from build123d import *

# Parameters (mm, degrees)
SKETCH_1_W          = 143
SKETCH_1_H          = 196
SKETCH_1_W_2        = 62
SKETCH_1_H_2        = 142
EXTRUDE_1_DEPTH     = 20
FILLET_1_R          = 12
SKETCH_2_R          = 3
CUT_EXTRUDE_1_DEPTH = 40
SKETCH_3_R          = 5
CUT_EXTRUDE_2_DEPTH = 40


with BuildPart() as part:
    # 草图1 → 凸台-拉伸1 (new, symmetric)
    with BuildSketch(Plane(origin=(0, 0, 0), x_dir=(1, 0, 0), z_dir=(0, 1, 0))):
        Rectangle(SKETCH_1_W, SKETCH_1_H)
        Rectangle(SKETCH_1_W_2, SKETCH_1_H_2, mode=Mode.SUBTRACT)
    extrude(amount=EXTRUDE_1_DEPTH, both=True)

    # 圆角1
    fillet_1_edges = [part.edges().sort_by_distance(p)[0] for p in [
        (-71.5, 0, -98),
        (71.5, 0, -98),
        (71.5, 0, 98),
        (-71.5, 0, 98),
    ]]
    fillet(fillet_1_edges, radius=FILLET_1_R)

    # 草图2 → 切除-拉伸1 (cut)
    with BuildSketch(Plane(origin=(0, 20, 0), x_dir=(1, 0, 0), z_dir=(0, 1, 0))):
        with Locations((-31, 71)):
            Circle(SKETCH_2_R)
        with Locations((31, 71)):
            Circle(SKETCH_2_R)
        with Locations((31, -71)):
            Circle(SKETCH_2_R)
        with Locations((-31, -71)):
            Circle(SKETCH_2_R)
    extrude(amount=-CUT_EXTRUDE_1_DEPTH, mode=Mode.SUBTRACT)

    # 草图3 → 切除-拉伸2 (cut)
    with BuildSketch(Plane(origin=(0, 20, 0), x_dir=(1, 0, 0), z_dir=(0, 1, 0))):
        with Locations((-71.5, 0)):
            Circle(SKETCH_3_R)
        with Locations((71.5, 0)):
            Circle(SKETCH_3_R)
    extrude(amount=-CUT_EXTRUDE_2_DEPTH, mode=Mode.SUBTRACT)


solid = part.part
The listing builds one solid part. Answer for the finished solid, in the listing's coordinates (mm). A direction names the side the tool comes from. Coordinates: 2 decimals unless noted, no trailing zeros. Loops run counter-clockwise (first coordinate to the right, second up) from the corner with the lowest first, then second, coordinate; pieces in that order, holes last. Notation, with made-up numbers: (52.5, 55.5) -> (75.5, 55.5) arc R5 cw to (75.5, 59.5) -> close; hole circle Ø10 at (26.25, 89). An arc over 180 degrees is marked (long way). Write item = value, one per line. Start each with the question number.
1) A cutting plane is placed at C-C (y = 13). Give the vertices of the cut face in (x, z), then the cut area to 3 significant figures.
2) A cutting plane is placed at A-A (z = -51). Give the vertices of the cut face in (x, y), then the cut area to 3 significant figures.
3) A cutting plane is placed at B-B (x = -19). Give the vertices of the cut face in (y, z), then the cut area to 3 significant figures.
4) The mould has two halves that part along X. Classify faces 3 (the face through (66.5, 0.3, -0.1)), 4 (the face through (-68.08, -0.28, -94.39)), 5 (the face through (-33.19, 0.28, 73.05)): released by +X, released by -X, zero draft, split by the parting line, or undercut.
5) A tool of negligible diameter and unlimited length cuts with its end or side. For faces 1 (the face through (-1, 0, -98)), 2 (the face through (0, 0, 71)), from which of +Z, -Z, +X, -X, +Y, -Y can it reach the whole face along a straight path? Write none if from no direction.
6) Straight lines are drawn through the part: line 1 (X direction, y = -3, z = 37.5); line 2 (Z direction, x = -13.5, y = 0); line 3 (Z direction, x = 29, y = 10). For each, find the intervals that lie inside material, in ascending order. Write a range as from..to.
Responses:
q1.outline = (-71.5, -86) arc R12 ccw to (-59.5, -98) -> (59.5, -98) arc R12 ccw to (71.5, -86) -> (71.5, -5) arc R5 cw to (71.5, 5) -> (71.5, 86) arc R12 ccw to (59.5, 98) -> (-59.5, 98) arc R12 ccw to (-71.5, 86) -> (-71.5, 5) arc R5 cw to (-71.5, -5) -> close; hole (-31, -68) arc R3 ccw (long way) to (-28, -71) -> (28, -71) arc R3 ccw (long way) to (31, -68) -> (31, 68) arc R3 ccw (long way) to (28, 71) -> (-28, 71) arc R3 ccw (long way) to (-31, 68) -> close
q1.area = 18,900 mm²
q2.outline = (-71.5, -20) -> (-31, -20) -> (-31, 20) -> (-71.5, 20) -> close; (31, -20) -> (71.5, -20) -> (71.5, 20) -> (31, 20) -> close
q2.area = 3,240 mm²
q3.outline = (-20, -98) -> (20, -98) -> (20, -71) -> (-20, -71) -> close; (-20, 71) -> (20, 71) -> (20, 98) -> (-20, 98) -> close
q3.area = 2,160 mm²
q4.face_3 = released by +X
q4.face_4 = released by -X
q4.face_5 = undercut
q5.face_1 = -Z, +X, -X, +Y, -Y
q5.face_2 = +Y, -Y
q6.line_1 = -71.5..-31, 31..71.5
q6.line_2 = -98..-71, 71..98
q6.line_3 = -98..-73.24, 73.24..98
